The listing builds one solid part. Answer for the finished solid, in the listing's coordinates (mm). A direction names the side the tool comes from. Coordinates: 2 decimals unless noted, no trailing zeros. Write each loop counter-clockwise with the first axis right and the second up, starting at its lowest first coordinate (ties: lowest second). Pieces come first, ordered by that corner, then holes.
from build123d import *

# Parameters (mm, degrees)
F0_W     = 377.952
F0_H     = 291.084
F1_DEPTH = 19.05
F2_W     = 333.375
F2_H     = 266.7
F3_DEPTH = 457.2
F4_W     = 307.975
F4_H     = 431.8
F5_DEPTH = 254
F6_W     = 307.975
F6_H     = 431.8
F7_DEPTH = 6.35


with BuildPart() as f1:
    # F0 (on Front) → F1 (new body)
    with BuildSketch(Plane.XZ):
        Rectangle(F0_W, F0_H)
    extrude(amount=F1_DEPTH)

    # F2 (on face) → F3 (join)
    with BuildSketch(Plane(origin=(0, 0, 0), x_dir=(-1, 0, 0), z_dir=(0, 1, 0))):
        Rectangle(F2_W, F2_H)
    extrude(amount=F3_DEPTH)

    # F4 (on face) → F5 (cut)
    with BuildSketch(Plane.XY.offset(133.35)):
        with Locations((0, 228.6)):
            Rectangle(F4_W, F4_H)
    extrude(amount=-F5_DEPTH, mode=Mode.SUBTRACT)

    # F6 (on face) → F7 (cut)
    with BuildSketch(Plane(origin=(0, 0, -133.35), x_dir=(1, 0, 0), z_dir=(0, 0, -1))):
        with Locations((0, -228.6)):
            Rectangle(F6_W, F6_H)
    extrude(amount=-F7_DEPTH, mode=Mode.SUBTRACT)


solid = f1.part
Q1. Determine the mould class of faces 1 (the face through (188.976, -9, -2)), 2 (the face through (-2, 444.5, 8)), 3 (the face through (-3, -9, -145.542)) for opening direction X: released by +X, released by -X, zero draft, split by the parting line, or undercut.
Answers below:
face 1: released by +X
face 2: undercut
face 3: zero draft
Q2. Find the intervals of material crossed by probe 1 along Y at (x, z) = (-106, 2); probe 2 along X at (y, z) = (295.5, 60.5); probe 3 along Z at (x, y) = (159, 319.5), in increasing order.
Answers below:
probe 1: y = -19.05 to 12.7, 444.5 to 457.2
probe 2: x = -166.69 to -153.99, 153.99 to 166.69
probe 3: z = -133.35 to 133.35
Q3. The part is cut by section C-C, the plane z = 126. Write down the section's boundary in (x, y).
Answers below:
outline: (-188.98, -19.05) - (188.98, -19.05) - (188.98, 0) - (166.69, 0) - (166.69, 457.2) - (-166.69, 457.2) - (-166.69, 0) - (-188.98, 0) - close; hole (-153.99, 12.7) - (153.99, 12.7) - (153.99, 444.5) - (-153.99, 444.5) - close
Q4. Given pin 1 (10 mm diameter, centred on y = 265, z = -13, fed in from -X); pin 2 (1.9 mm diameter, centred on y = 335.5, z = -130.5, fed in from +X); pin 3 (5 mm diameter, centred on x = 56, y = 37.5, fed in from -Z), each flat-ended and moving along its own axis, determine where each tip first touches the part or whether it passes through.
Answers below:
pin 1: stops at x = -166.69
pin 2: stops at x = 166.69
pin 3: stops at z = -127
Q5. The part is cut by section B-B, the plane y = 424. Write down the section's boundary in (x, z).
Answers below:
outline: (-166.69, -133.35) - (-153.99, -133.35) - (-153.99, -127) - (153.99, -127) - (153.99, -133.35) - (166.69, -133.35) - (166.69, 133.35) - (153.99, 133.35) - (153.99, -120.65) - (-153.99, -120.65) - (-153.99, 133.35) - (-166.69, 133.35) - close
Q6. The part is cut by section A-A, the plane x = 51. Write down the section's boundary in (y, z), then the cut area to 3 significant figures.
Answers below:
outline: (-19.05, -145.54) - (0, -145.54) - (0, -133.35) - (12.7, -133.35) - (12.7, -127) - (444.5, -127) - (444.5, -133.35) - (457.2, -133.35) - (457.2, 133.35) - (444.5, 133.35) - (444.5, -120.65) - (12.7, -120.65) - (12.7, 133.35) - (0, 133.35) - (0, 145.54) - (-19.05, 145.54) - close
area: 15,100 mm2
Q7. Which of the six approach directions +Z, -Z, +X, -X, +Y, -Y give full straight-line access (tool end or side, diameter ignored) to faces 4 (the face through (161, 228, 133.35)), 5 (the face through (-166.688, 225, -2)), 6 (the face through (161, 228, -133.35)), 7 (the face through (-153.988, 226, 8))?
Answers below:
face 4: +Z, +X, -X, +Y
face 5: +Z, -Z, -X, +Y
face 6: -Z, +X, -X, +Y
face 7: +Z
